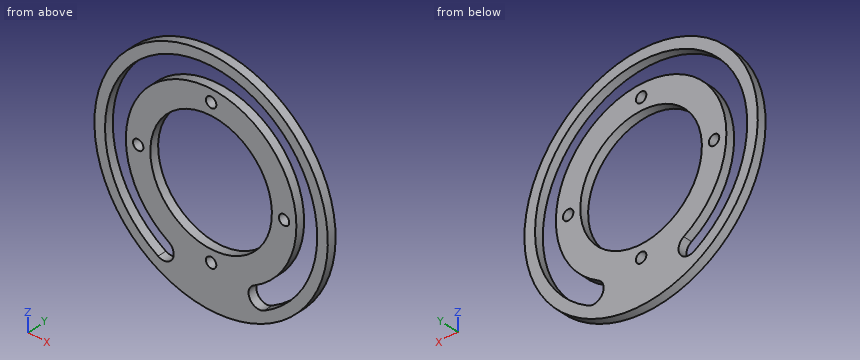
from build123d import *

# Parameters (mm, degrees)
SKETCH1_R           = 42.672
SKETCH1_R_2         = 22.225
SKETCH1_R_3         = 1.905
BOSS_EXTRUDE1_DEPTH = 3.175
CUT_EXTRUDE1_DEPTH  = 61.430785143


with BuildPart() as part:
    # Sketch1 → Boss-Extrude1 (new body)
    with BuildSketch(Plane(origin=(0, 0, 0), x_dir=(1, 0, 0), z_dir=(0, 1, 0))):
        with Locations(Location((0, 0, 0), (0, 0, 270))):
            Circle(SKETCH1_R)
        with Locations(Location((0, 0, 0), (0, 0, 270))):
            Circle(SKETCH1_R_2, mode=Mode.SUBTRACT)
        with Locations(Location((0, 26.67, 0), (0, 0, 270))):
            Circle(SKETCH1_R_3, mode=Mode.SUBTRACT)
        with Locations(Location((26.67, 0, 0), (0, 0, 270))):
            Circle(SKETCH1_R_3, mode=Mode.SUBTRACT)
        with Locations(Location((0, -26.67, 0), (0, 0, 270))):
            Circle(SKETCH1_R_3, mode=Mode.SUBTRACT)
        with Locations(Location((-26.67, 0, 0), (0, 0, 270))):
            Circle(SKETCH1_R_3, mode=Mode.SUBTRACT)
    extrude(amount=BOSS_EXTRUDE1_DEPTH)

    # Sketch2 → Cut-Extrude1 (cut, through all)
    with BuildSketch(Plane(origin=(0, 3.175, 0), x_dir=(1, 0, 0), z_dir=(0, 1, 0))):
        with BuildLine():
            ThreePointArc((-15.58925, 27.001373052), (-14.194693212, 32.20592984), (-19.39925, 33.600486629))
            ThreePointArc((-19.39925, 33.600486629), (0, -38.7985), (19.39925, 33.600486629))
            ThreePointArc((19.39925, 33.600486629), (14.194693212, 32.20592984), (15.58925, 27.001373052))
            ThreePointArc((15.58925, 27.001373052), (0, -31.1785), (-15.58925, 27.001373052))
        make_face()
    extrude(amount=-CUT_EXTRUDE1_DEPTH, mode=Mode.SUBTRACT)


solid = part.part
Geometry check sheet. Reference: the model listing, model coordinates, mm. Coordinates: 2 decimals unless noted, no trailing zeros. Loops run counter-clockwise (first coordinate to the right, second up) from the corner with the lowest first, then second, coordinate; pieces in that order, holes last. Notation, with made-up numbers: (22.25, -21.5) - (27.25, -21.5) arc R13 cw to (27.25, -16.5) - close; hole circle Ø1 at (81.25, 65.25). An arc over 180 degrees is marked (long way). Use one line per item in the form item = value. Start each with the question number.
Item 1: Thickness scan on probe 1 along X at (y, z) = (1.7, 0) (1 decimal); probe 2 along Z at (x, y) = (25, 0.7); probe 3 along Z at (x, y) = (-3.5, 1.3). Record the ranges inside material, lowest first.
Item 2: Section check C-C, the plane z = -11.5. Enter the section's corners in (x, y) (3 decimals), and give its area (3 significant figures).
Item 3: Section check B-B, the plane z = 0. Enter the section's corners in (x, y) (1 decimal), and give its area (3 significant figures).
Item 4: Section check D-D, the plane y = 1.1. Give the number of separate pieces and of enclosed holes in the cut face, and give its area (3 significant figures).
Item 5: Section check A-A, the plane x = 0. Enter the section's corners in (y, z) (1 decimal), and give its area (3 significant figures).
Item 6: Gauge pin test, flat ends, axial feed: pin 1 (1.5 mm diameter, centred on x = 31, y = 2.5, fed in from -Z); pin 2 (4.5 mm diameter, centred on x = 0, z = 26.67, fed in from -Y); pin 3 (1.5 mm diameter, centred on y = 1.5, z = -2.5, fed in from -X). Record the tip position at first contact, or that the pin passes through.
Computed:
q1.probe_1 = -42.7 to -38.8, -31.2 to -28.6, -24.8 to -22.2, 22.2 to 24.8, 28.6 to 31.2, 38.8 to 42.7
q1.probe_2 = -34.58 to -29.67, -18.63 to -0.92, 0.92 to 18.63, 29.67 to 34.58
q1.probe_3 = -42.53 to -21.95, 21.95 to 30.98, 38.64 to 42.53
q2.outline = (-41.093, 0) - (-37.055, 0) - (-37.055, 3.175) - (-41.093, 3.175) - close; (-28.98, 0) - (-19.018, 0) - (-19.018, 3.175) - (-28.98, 3.175) - close; (19.018, 0) - (28.98, 0) - (28.98, 3.175) - (19.018, 3.175) - close; (37.055, 0) - (41.093, 0) - (41.093, 3.175) - (37.055, 3.175) - close
q2.area = 88.9 mm2
q3.outline = (-42.7, 0) - (-38.8, 0) - (-38.8, 3.2) - (-42.7, 3.2) - close; (-31.2, 0) - (-28.6, 0) - (-28.6, 3.2) - (-31.2, 3.2) - close; (-24.8, 0) - (-22.2, 0) - (-22.2, 3.2) - (-24.8, 3.2) - close; (22.2, 0) - (24.8, 0) - (24.8, 3.2) - (22.2, 3.2) - close; (28.6, 0) - (31.2, 0) - (31.2, 3.2) - (28.6, 3.2) - close; (38.8, 0) - (42.7, 0) - (42.7, 3.2) - (38.8, 3.2) - close
q3.area = 57.3 mm2
q4.separate_pieces = 1
q4.enclosed_holes = 6
q4.area = 2,680 mm2
q5.outline = (0, -42.7) - (3.2, -42.7) - (3.2, -28.6) - (0, -28.6) - close; (0, -24.8) - (3.2, -24.8) - (3.2, -22.2) - (0, -22.2) - close; (0, 22.2) - (3.2, 22.2) - (3.2, 24.8) - (0, 24.8) - close; (0, 28.6) - (3.2, 28.6) - (3.2, 31.2) - (0, 31.2) - close; (0, 38.8) - (3.2, 38.8) - (3.2, 42.7) - (0, 42.7) - close
q5.area = 81.5 mm2
q6.pin_1 = -30.1
q6.pin_2 = 0
q6.pin_3 = -42.64
